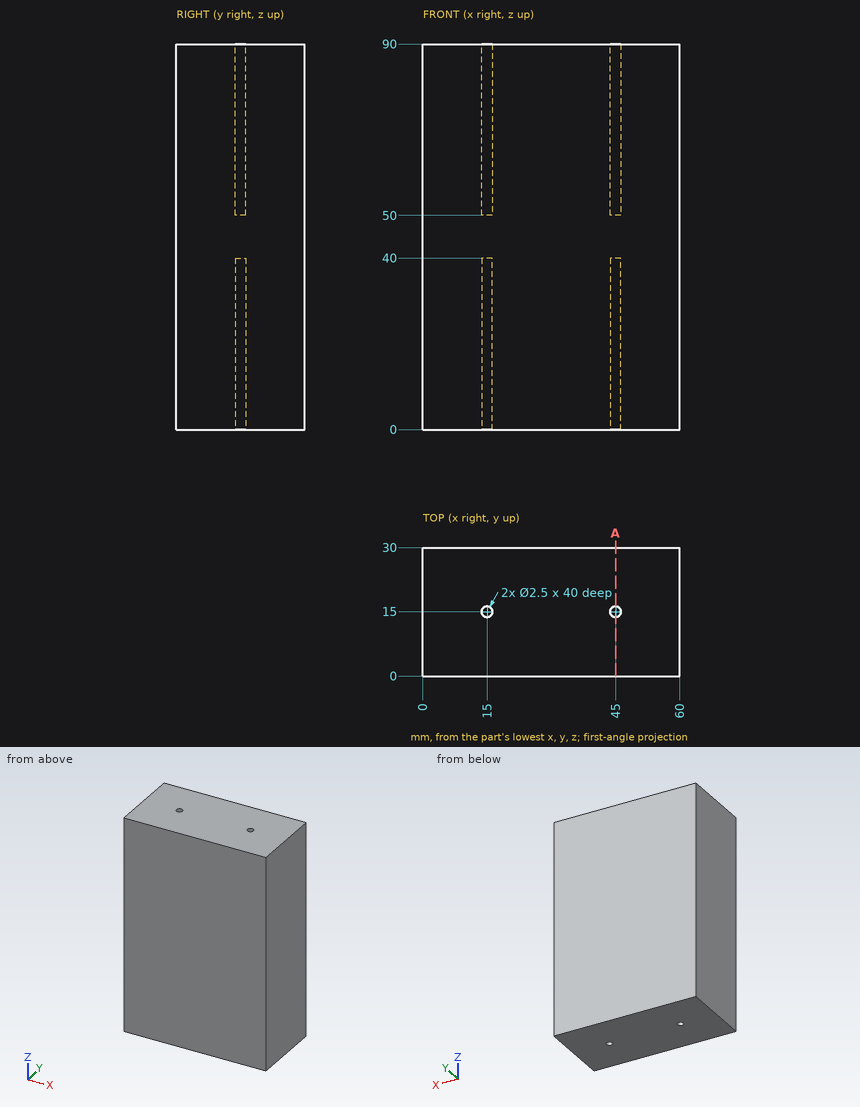
Source: three-view drawing plus pictorial views. Frame: mm from the lowest corner of the part. Give positions to 0.01 mm unless a question says otherwise; leave off trailing zeros. Write each loop counter-clockwise with the first axis right and the second up, starting at its lowest first coordinate (ties: lowest second). Pieces come first, ordered by that corner, then holes. Notation, with made-up numbers: M 18,-32.75 L 59,-32.75 A13 ccw 59,-28.75 Z; hole C 82,-3 d4. An arc over 180 degrees is marked long. Use one line per item in the form item = value.
1. Ray query, L1, parallel to X at y = 15, z = 21; L2, parallel to Y at x = 45, z = 27; L3, parallel to X at y = 16, z = 39.5. Return the intervals inside material, ascending.
Outcome:
L1 = 0 to 13.75, 16.25 to 43.75, 46.25 to 60
L2 = 0 to 13.75, 16.25 to 30
L3 = 0 to 14.25, 15.75 to 44.25, 45.75 to 60
2. First-contact query: P1, Ø2, axis at x = 45, y = 15, coming from the -Z side. Flat tip, straight axial feed; report the tip coordinate or a pass-through.
Outcome:
P1 = 40
3. Cut plane A-A on x = 45. Return loops of the section in (y, z).
Outcome:
outline = M 0,0 L 13.75,0 L 13.75,40 L 16.25,40 L 16.25,0 L 30,0 L 30,90 L 16.25,90 L 16.25,50 L 13.75,50 L 13.75,90 L 0,90 Z
